The model under review builds one solid part; all positions refer to its coordinate system, in mm. Face numbers are marked on the shaded views. A direction names the side the tool comes from. Give positions to 0.01 mm unless a question says otherwise; leave off trailing zeros. Order: outer loops, then holes, each group sorted by start corner. A loop starts at its lowest first (then second) coordinate and runs counter-clockwise, first axis right, second up. Notation, with made-up numbers: (-12.75, -32.5) - (-1.75, -32.5) arc R36 ccw to (-1.75, 5.5) - close; hole circle Ø10 at (41.5, 3.5). An arc over 180 degrees is marked (long way). Use CSV: the item, a comma, the result in double quotes.
Autodesk Inventor part; units mm, degrees
ref_plane "YZ Plane" through (0, 0, 0) normal (1, 0, 0) x (0, 1, 0)
ref_plane "XZ Plane" through (0, 0, 0) normal (0, 1, 0) x (-1, 0, 0)
ref_plane "XY Plane" through (0, 0, 0) normal (0, 0, 1) x (1, 0, 0)
sketch "Sketch2" plane through (0, 0, 0) normal (0, 0, 1) x (1, 0, 0)
  line L0 (-9.4794, 5.5186) -> (11.8294, 5.5186)
  circle A0 centre (-6.0645, -2.4947) radius 1.05
  circle A1 centre (8.4145, -2.4947) radius 1.05
  circle A2 centre (8.4145, 1.6737) radius 1.05
  circle A3 centre (-6.0645, 1.6737) radius 1.05
  line L1 (-9.4794, 5.5186) -> (-9.4794, -157.7914)
  line L2 (11.8294, -157.7914) -> (11.8294, 5.5186)
  line L3 (-9.4794, -157.7914) -> (-9.4794, -161.9314)
  line L4 (-9.4794, -161.9314) -> (11.8294, -161.9314)
  line L5 (11.8294, -161.9314) -> (11.8294, -157.7914)
  point P0 (0, 0)
  dimension "d20" = 163.31
  dimension "d31" = 4.14
  dimension "d37" = 2.1
  dimension "d38" = 2.1
  dimension "d39" = 2.1
  dimension "d40" = 2.1
extrude "Extrusion1" add sketch "Sketch2" along normal blind 2
fillet "Fillet6" radius 0.5 2 edges at (11.8294, 5.5186, 1) (-9.4794, 5.5186, 1)
sketch "Sketch9" plane through (0, 0, 2) normal (0, 0, 1) x (1, 0, 0)
  line L0 (-9.4794, -161.9314) -> (11.8294, -161.9314)
  line L1 (-9.4794, -161.9314) -> (11.8294, -161.9314)
  line L2 (11.8294, -161.9314) -> (11.8294, -159.9314)
  line L3 (11.8294, -159.9314) -> (-9.4794, -159.9314)
  line L4 (-9.4794, -159.9314) -> (-9.4794, -161.9314)
  point P0 (0, 0)
  dimension "d32" = 2
extrude "Extrusion7" add sketch "Sketch9" along normal blind 30
sketch "Sketch10" plane through (-9.4794, -159.9314, 2) normal (0, 1, 0) x (1, 0, 0)
  point P0 (9.4794, 2)
fillet "Fillet10" radius 0.5 2 edges at (1.175, -159.9314, 2) (1.175, -161.9314, 0)
fillet "Fillet11" radius 0.5 2 edges at (-9.4794, -160.9314, 32) (11.8294, -160.9314, 32)
properties part number "Bracket Holder" material "Aluminum 6061"
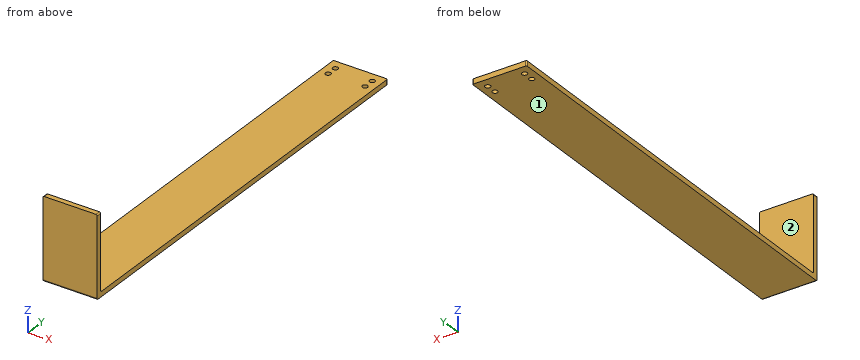
Item 1: Tool access review of the marked faces 1 and 2: name each direction out of +Z, -Z, +X, -X, +Y, -Y from which nothing blocks a thin tool from reaching the whole face with its end or side.
Results list:
face 1,"-Z, +X, -X, +Y, -Y"
face 2,"+Z, +X, -X, +Y"
Item 2: Take a section at B-B, the plane z = 4. Give the boundary of the cut face in (x, y), and give its area (3 significant figures).
Results list:
outline,"(-9.48, -161.93) - (11.83, -161.93) - (11.83, -159.93) - (-9.48, -159.93) - close"
area,"42.6 mm2"
Item 3: Clearance check with flat-ended pins moving along their axes: pin 1 (1.5 mm diameter, centred on x = 9.5, z = 5.5, fed in from +Y); pin 2 (1 mm diameter, centred on x = 2.5, y = -134, fed in from -Z); pin 3 (10.5 mm diameter, centred on x = -2, y = -107.5, fed in from +Z). State where each tip first meets the part, or that it passes through.
Results list:
pin 1,"stops at y = -159.93"
pin 2,"stops at z = 0"
pin 3,"stops at z = 2"
Item 4: Wall thickness on L1, parallel to Z at x = 2, y = -135; L2, parallel to Y at x = 0.75, z = 21: over which ranges is each line inside the solid? List them lowest first.
Results list:
L1,"z = 0 to 2"
L2,"y = -161.93 to -159.93"
Item 5: Take a section at C-C, the plane y = -118.5. Give the boundary of the cut face in (x, z).
Results list:
outline,"(-9.48, 0) - (11.83, 0) - (11.83, 2) - (-9.48, 2) - close"
Item 6: Take a section at A-A, the plane x = 2.25. Give the boundary of the cut face in (y, z).
Results list:
outline,"(-161.93, 0.5) arc R0.5 ccw to (-161.43, 0) - (5.52, 0) - (5.52, 2) - (-159.43, 2) arc R0.5 cw to (-159.93, 2.5) - (-159.93, 32) - (-161.93, 32) - close"
